```python
from build123d import *

# Parameters (mm, degrees)
SKETCH1_W           = 50
SKETCH1_H           = 50
SKETCH1_R           = 1.5
BOSS_EXTRUDE1_DEPTH = 3
BOSS_EXTRUDE2_DEPTH = 75
CUT_EXTRUDE1_DEPTH  = 96.963534741
SKETCH4_W           = 50
SKETCH4_H           = 70.710678118
BOSS_EXTRUDE3_DEPTH = 5


with BuildPart() as part:
    # Sketch1 → Boss-Extrude1 (new body)
    with BuildSketch(Plane(origin=(0, 0, 0), x_dir=(1, 0, 0), z_dir=(0, 1, 0))):
        Rectangle(SKETCH1_W, SKETCH1_H)
        with Locations(Location((-20, -20, 0), (0, 0, 270))):
            Circle(SKETCH1_R, mode=Mode.SUBTRACT)
        with Locations(Location((-20, 20, 0), (0, 0, 270))):
            Circle(SKETCH1_R, mode=Mode.SUBTRACT)
        with Locations(Location((20, 20, 0), (0, 0, 270))):
            Circle(SKETCH1_R, mode=Mode.SUBTRACT)
        with Locations(Location((20, -20, 0), (0, 0, 270))):
            Circle(SKETCH1_R, mode=Mode.SUBTRACT)
    extrude(amount=BOSS_EXTRUDE1_DEPTH)

    # Sketch2 → Boss-Extrude2 (add)
    with BuildSketch(Plane(origin=(0, 3, 0), x_dir=(1, 0, 0), z_dir=(0, 1, 0))):
        Polygon((0, 25), (-25, 0), (0, -25), (25, 0), align=None)
        Polygon((0, 17.928932188), (-17.928932188, 0), (0, -17.928932188), (17.928932188, 0), align=None, mode=Mode.SUBTRACT)
    extrude(amount=BOSS_EXTRUDE2_DEPTH)

    # Sketch3 → Cut-Extrude1 (cut, through all)
    with BuildSketch(Plane.XY.offset(25)):
        Polygon((25, 78), (-25, 78), (-25, 28), align=None)
    extrude(amount=-CUT_EXTRUDE1_DEPTH, mode=Mode.SUBTRACT)

    # Sketch4 → Boss-Extrude3 (add, along a direction that is not the sketch's normal)
    with BuildSketch(Plane(origin=(-26.5, 26.5, 0), x_dir=(0, 0, 1), z_dir=(-0.7071067811865438, 0.7071067811865513, 0))):
        with Locations((0, 37.476659403)):
            Rectangle(SKETCH4_W, SKETCH4_H)
        Polygon((-17.928932188, 37.476659403), (0, 62.831998462), (17.928932188, 37.476659403), (0, 12.121320344), align=None, mode=Mode.SUBTRACT)
    extrude(amount=BOSS_EXTRUDE3_DEPTH, dir=(0, 1, 0))


solid = part.part
```
Part model, mm, in its own coordinate system. A direction names the side the tool comes from. Round coordinates to 2 decimals unless told otherwise and drop trailing zeros. Write each loop counter-clockwise with the first axis right and the second up, starting at its lowest first coordinate (ties: lowest second). Pieces come first, ordered by that corner, then holes.
Item 1: Drop flat-ended pins along their axis: pin 1 Ø5 at (x, z) = (11, -4) entering from -Y; pin 2 Ø12.5 at (x, z) = (-18, -8) entering from +Y; pin 3 Ø5 at (x, y) = (14.5, 50) entering from -Z; pin 4 Ø7.5 at (x, z) = (-11.5, 17.5) entering from +Y. Give the stop position or say it passes through.
Results:
pin 1: stops at y = 0
pin 2: stops at y = 46.25
pin 3: stops at z = -13
pin 4: stops at y = 50.25
Item 2: Two-plate mould, pull along X, no slides. Class faces 4 (the cylindrical face through (-18.99, 1.48, 18.89)), 5 (the flat face through (-25, 1, 0)), 6 (the flat face through (15, 68, -15)), 7 (the cylindrical face through (-18.99, 1.48, -21.11)): +X half, -X half, draft (parallel to the pull), parting line (faces both ways), or undercut.
Results:
face 4: undercut
face 5: -X half
face 6: +X half
face 7: undercut
Item 3: Which spindle directions (+Z, -Z, +X, -X, +Y, -Y) get a long thin tool onto all of the face, cutting with end or side? Do faces 1 (the flat face through (-15, 3, -15)), 2 (the flat face through (0, 3, 0)), 3 (the flat face through (-12, 22, -13)). Say none if no direction does.
Results:
face 1: -Z, -X
face 2: +Y
face 3: -Z
Item 4: Probe L1, parallel to X at y = 2.25, z = -20; L2, parallel to Y at x = -12, z = 5.5; L3, parallel to Y at x = 22.5, z = 17. List the from-to ranges inside material, lowest first.
Results:
L1: x = -25 to -21.5, -18.5 to 18.5, 21.5 to 25
L2: y = 0 to 3
L3: y = 0 to 3, 75.5 to 80.5
Item 5: Cut at A-A, the plane x = 20. Give the cut face in (y, z), plus the area to 3 significant figures.
Results:
outline: (0, -25) - (3, -25) - (3, -21.5) - (0, -21.5) - close; (0, -18.5) - (3, -18.5) - (3, -5) - (73, -5) - (73, -25) - (78, -25) - (78, 25) - (73, 25) - (73, 5) - (3, 5) - (3, 18.5) - (0, 18.5) - close; (0, 21.5) - (3, 21.5) - (3, 25) - (0, 25) - close
area: 1,080 mm2
Item 6: Cut at D-D, the plane x = 11.5. Give the cut face in (y, z).
Results:
outline: (0, -25) - (3, -25) - (3, -13.5) - (64.5, -13.5) - (64.5, -25) - (69.5, -25) - (69.5, -6.43) - (3, -6.43) - (3, 6.43) - (69.5, 6.43) - (69.5, 25) - (64.5, 25) - (64.5, 13.5) - (3, 13.5) - (3, 25) - (0, 25) - close
Item 7: Cut at C-C, the plane y = 26. Give the cut face in (x, z), plus the area to 3 significant figures.
Results:
outline: (-25, 0) - (0, -25) - (25, 0) - (0, 25) - close; hole (-17.93, 0) - (0, -17.93) - (17.93, 0) - (0, 17.93) - close
area: 607 mm2
Item 8: Cut at B-B, the plane z = 20. Give the cut face in (x, y).
Results:
outline: (-25, 0) - (-21.5, 0) - (-21.5, 3) - (-25, 3) - close; (-25, 28) - (-5, 48) - (-5, 3) - (-18.5, 3) - (-18.5, 0) - (18.5, 0) - (18.5, 3) - (5, 3) - (5, 58) - (25, 78) - (25, 83) - (-25, 33) - close; (21.5, 0) - (25, 0) - (25, 3) - (21.5, 3) - close
